```python
from build123d import *

# Parameters (mm, degrees)
ESQUISSE1_R             = 16.5
ESQUISSE1_R_2           = 14.29
BOSS_EXTRU_1_DEPTH      = 6
BOSS_EXTRU_2_START      = 10
ESQUISSE2_R             = 16.5
BOSS_EXTRU_2_DEPTH      = 10
BOSS_EXTRU_3_DEPTH      = 5
BOSS_EXTRU_4_DEPTH      = 16
ESQUISSE7_R             = 2
ESQUISSE7_W             = 60
ESQUISSE7_H             = 4
ENL_V_MAT_EXTRU_1_DEPTH = 57.071383076
ESQUISSE8_R             = 7.5
ENL_V_MAT_EXTRU_2_DEPTH = 39.23937761
ESQUISSE10_W            = 60
ESQUISSE10_H            = 5
BOSS_EXTRU_5_DEPTH      = 5
ENL_V_MAT_EXTRU_4_DEPTH = 5


with BuildPart() as part:
    # Esquisse1 → Boss.-Extru.1 (new body)
    with BuildSketch(Plane.XY):
        Circle(ESQUISSE1_R)
        Circle(ESQUISSE1_R_2, mode=Mode.SUBTRACT)
    extrude(amount=BOSS_EXTRU_1_DEPTH)

    # Esquisse2 → Boss.-Extru.2 (add)
    with BuildSketch(Plane(origin=(0, 0, 0), x_dir=(-1, 0, 0), z_dir=(0, 0, -1)).offset(BOSS_EXTRU_2_START)):
        Circle(ESQUISSE2_R)
    extrude(amount=-BOSS_EXTRU_2_DEPTH)



with BuildPart() as body_2:
    # Esquisse3 → Boss.-Extru.3 (new body)
    with BuildSketch(Plane(origin=(0, 16.5, 0), x_dir=(1, 0, 0), z_dir=(0, 1, 0))):
        Polygon((0, 10), (40, 10), (40, -10), (0, -10), (-40, -10), (-40, 10), align=None)
    extrude(amount=BOSS_EXTRU_3_DEPTH)


with BuildPart() as part_1:
    add(part.part)

    add(body_2.part)  # Boss.-Extru.4 merges body 2
    # Esquisse4 → Boss.-Extru.4 (add)
    with BuildSketch(Plane.XY.offset(-10)):
        with BuildLine():
            ThreePointArc((-16.5, 0), (-11.66726189, 11.66726189), (0, 16.5))
            Line((0, 16.5), (-16.5, 16.5))
            Line((-16.5, 16.5), (-16.5, 0))
        make_face()
        with BuildLine():
            ThreePointArc((16.5, 0), (11.66726189, 11.66726189), (0, 16.5))
            Line((0, 16.5), (16.5, 16.5))
            Line((16.5, 16.5), (16.5, 0))
        make_face()
    extrude(amount=BOSS_EXTRU_4_DEPTH)

    # Esquisse7 → Enlèv. mat.-Extru.1 (cut, through all)
    with BuildSketch(Plane(origin=(0, 21.5, 0), x_dir=(1, 0, 0), z_dir=(0, 1, 0))):
        Polygon((-40, -10), (-30, -10), (-30, -6), (-30, 10), (-40, 10), align=None)
        Polygon((30, -6), (30, -10), (40, -10), (40, 10), (30, 10), align=None)
        with Locations((22.5, 10)):
            Circle(ESQUISSE7_R)
        with Locations((-22.5, 10)):
            Circle(ESQUISSE7_R)
        with Locations((0, -8)):
            Rectangle(ESQUISSE7_W, ESQUISSE7_H)
    extrude(amount=-ENL_V_MAT_EXTRU_1_DEPTH, mode=Mode.SUBTRACT)

    # Esquisse8 → Enlèv. mat.-Extru.2 (cut, through all)
    with BuildSketch(Plane.XY):
        Circle(ESQUISSE8_R)
    extrude(amount=-ENL_V_MAT_EXTRU_2_DEPTH, mode=Mode.SUBTRACT)

    # Esquisse10 → Boss.-Extru.5 (add)
    with BuildSketch(Plane(origin=(0, 0, -10), x_dir=(-1, 0, 0), z_dir=(0, 0, -1))):
        with Locations((0, 19)):
            Rectangle(ESQUISSE10_W, ESQUISSE10_H)
    extrude(amount=BOSS_EXTRU_5_DEPTH)

    # Esquisse11 → Enlèv. mat.-Extru.4 (cut)
    with BuildSketch(Plane(origin=(0, 21.5, 0), x_dir=(1, 0, 0), z_dir=(0, 1, 0))):
        Polygon((-18, -6), (-30, 4.5), (-30, -6), align=None)
        Polygon((30, 4.5), (18, -6), (30, -6), align=None)
        with BuildLine():
            Line((20.5, 10), (24.5, 10))
            ThreePointArc((24.5, 10), (22.5, 12), (20.5, 10))
        make_face()
        with BuildLine():
            ThreePointArc((20.5, 10), (22.5, 8), (24.5, 10))
            Line((24.5, 10), (20.5, 10))
        make_face()
        with BuildLine():
            Line((-24.5, 10), (-20.5, 10))
            ThreePointArc((-20.5, 10), (-22.5, 12), (-24.5, 10))
        make_face()
        with BuildLine():
            ThreePointArc((-24.5, 10), (-22.5, 8), (-20.5, 10))
            Line((-20.5, 10), (-24.5, 10))
        make_face()
    extrude(amount=-ENL_V_MAT_EXTRU_4_DEPTH, mode=Mode.SUBTRACT)


solid = part_1.part
```
Verification items for the finished model (mm, model axes). A direction names the side the tool comes from. Round coordinates to 2 decimals unless told otherwise and drop trailing zeros. Write each loop counter-clockwise with the first axis right and the second up, starting at its lowest first coordinate (ties: lowest second). Pieces come first, ordered by that corner, then holes. Notation, with made-up numbers: (54.5, 52.25) -> (97.5, 52.25) arc R22 cw to (97.5, 71.25) -> close; hole circle Ø1 at (75.5, -20). An arc over 180 degrees is marked (long way). Write each question's results on one line, items separated by ' | '.
Q1. Sectioned sample at B-B, the plane y = 3. Record the boundary of the cut face in (x, z).
Derived:
outline: (-16.5, -10) -> (-6.87, -10) -> (-6.87, 0) -> (-13.97, 0) -> (-13.97, 6) -> (-16.5, 6) -> close; (6.87, -10) -> (16.5, -10) -> (16.5, 6) -> (13.97, 6) -> (13.97, 0) -> (6.87, 0) -> close
Q2. Sectioned sample at C-C, the plane z = 4. Record the boundary of the cut face in (x, y), and give its area (3 significant figures).
Derived:
outline: (-20.29, 16.5) -> (-16.5, 16.5) -> (-16.5, 0) arc R16.5 ccw to (16.5, 0) -> (16.5, 16.5) -> (20.29, 16.5) -> (20.29, 21.5) -> (-20.29, 21.5) -> close; hole circle Ø28.58 at (0, 0) | area: 533 mm²
Q3. Access from +Z, -Z, +X, -X, +Y, -Y to the whole of each face (thin tool, end or side, straight path). Record for faces 1 (the face through (16.5, 8, -2)), 2 (the face through (-16.5, 8, -2)), 3 (the face through (0, 8, -10)), 4 (the face through (0, 19, -15)), 5 (the face through (-6, -6, 0)).
Derived:
face 1: +Z, -Z, +X, -Y | face 2: +Z, -Z, -X, -Y | face 3: -Z, +X, -X, -Y | face 4: -Z, +X, -X, +Y, -Y | face 5: +Z
Q4. Sectioned sample at A-A, the plane x = 0. Record the boundary of the cut face in (y, z), and give its area (3 significant figures).
Derived:
outline: (-16.5, -10) -> (-7.5, -10) -> (-7.5, 0) -> (-14.29, 0) -> (-14.29, 6) -> (-16.5, 6) -> close; (7.5, -10) -> (16.5, -10) -> (16.5, -15) -> (21.5, -15) -> (21.5, 6) -> (14.29, 6) -> (14.29, 0) -> (7.5, 0) -> close | area: 312 mm²
Q5. Draft check along Z on faces 6 (the face through (-23.974, 19.035, -11.352)), 7 (the face through (0, 16.5, -11)), 8 (the face through (21.026, 19.035, -11.352)), 9 (the face through (-23.92, 19.04, 0.82)). Enter one of: released by +Z, released by -Z, zero draft, split by the parting line, or undercut.
Derived:
face 6: undercut | face 7: zero draft | face 8: undercut | face 9: released by +Z
Q6. Go/stop test with flat-tipped pins: pin 1 Ø4.5 at (x, z) = (-22.5, -10) entering from +Y; pin 2 Ø3 at (x, z) = (-4, -1.5) entering from -Y; pin 3 Ø3 at (x, z) = (8, 1.5) entering from -Y; pin 4 Ø17 at (x, y) = (0, 0) entering from +Z. Record where each tip stops, or that it passes through.
Derived:
pin 1: stops at y = 21.5 | pin 2: stops at y = -16.31 | pin 3: stops at y = -15.17 | pin 4: stops at z = 0
Q7. Thickness scan on probe 1 along X at (y, z) = (20.35, -10); probe 2 along X at (y, z) = (18, -8.75); probe 3 along X at (y, z) = (15, 4). Record the ranges inside material, lowest first.
Derived:
probe 1: x = -30 to -24.5, -20.5 to 20.5, 24.5 to 30 | probe 2: x = -30 to -24.06, -20.94 to 20.94, 24.06 to 30 | probe 3: x = -16.5 to 16.5
Q8. Sectioned sample at D-D, the plane x = -6. Record the boundary of the cut face in (y, z).
Derived:
outline: (-15.37, -10) -> (-4.5, -10) -> (-4.5, 0) -> (-12.97, 0) -> (-12.97, 6) -> (-15.37, 6) -> close; (4.5, -10) -> (16.5, -10) -> (16.5, -15) -> (21.5, -15) -> (21.5, 6) -> (12.97, 6) -> (12.97, 0) -> (4.5, 0) -> close
